The listing builds one solid part. Answer for the finished solid, in the listing's coordinates (mm). A direction names the side the tool comes from. Coordinates: 2 decimals unless noted, no trailing zeros. Write each loop counter-clockwise with the first axis right and the second up, starting at its lowest first coordinate (ties: lowest second). Pieces come first, ordered by that corner, then holes.
(1) The part is cut by section D-D on y = 3.5. Determine the outline of the cut face in (x, z).
(2) The part is cut by section C-C on x = 26. Determine the outline of the cut face in (y, z).
(3) For a pull along X with two mould halves and no side action, classify faces 1 (the flat face through (26, 0.5, 11)), 2 (the cylindrical face through (-28.747, 2.965, 5.121)), 3 (the cylindrical face through (0, 23, 11)) as +X half, -X half, draft (parallel to the pull), parting line (faces both ways), or undercut.
(4) Which of the six approach directions +Z, -Z, +X, -X, +Y, -Y give full straight-line access (tool end or side, diameter ignored) to faces 4 (the flat face through (-28, 5.5, 11)), 5 (the flat face through (28, 5.5, 11)), 6 (the cylindrical face through (0, 18, 11))?
(5) The part is cut by section B-B on y = 17. Determine the outline of the cut face in (x, z).
(6) Given P1, Ø6, axis at x = 29, z = 7.5, coming from the +Y side; P2, Ø12, axis at y = 20, z = 8, coming from the -X side; P3, Ø4.5, axis at x = -26, z = 18, coming from the -Y side; P4, Ø6.5, axis at x = 26, z = 5, coming from the -Y side, each flat-ended and moving along its own axis, determine where each tip first touches the part or whether it passes through.
(7) Straight lines are drawn through the part: line 1 (Z direction, x = -26, y = 2.95); line 2 (X direction, y = 4.5, z = 5.75); line 3 (X direction, y = 8.25, z = 15). For each, find the intervals that lie inside material, in ascending order.
from build123d import *

# Parameters (mm, degrees)
BOSS_EXTRUDE1_DEPTH = 23
SKETCH2_R           = 2.75
CUT_EXTRUDE1_DEPTH  = 47.810789355


with BuildPart() as part:
    # Sketch1 → Boss-Extrude1 (new body)
    with BuildSketch(Plane.XY):
        with BuildLine():
            Line((-17.993054215, 0.5), (-34, 0.5))
            Line((-34, 0.5), (-34, 5.5))
            Line((-34, 5.5), (-22.332711434, 5.5))
            ThreePointArc((-22.332711434, 5.5), (0, 23), (22.332711434, 5.5))
            Line((22.332711434, 5.5), (34, 5.5))
            Line((34, 5.5), (34, 0.5))
            Line((34, 0.5), (17.993054215, 0.5))
            ThreePointArc((17.993054215, 0.5), (0, 18), (-17.993054215, 0.5))
        make_face()
    extrude(amount=BOSS_EXTRUDE1_DEPTH)

    # Sketch2 → Cut-Extrude1 (cut, through all)
    with BuildSketch(Plane.XZ.offset(-0.5)):
        with Locations((-26, 18)):
            Circle(SKETCH2_R)
        with Locations((-26, 5)):
            Circle(SKETCH2_R)
        with Locations((26, 5)):
            Circle(SKETCH2_R)
        with Locations((26, 18)):
            Circle(SKETCH2_R)
    extrude(amount=-CUT_EXTRUDE1_DEPTH, mode=Mode.SUBTRACT)


solid = part.part
Model answer:
1. outline: (-34, 0) - (-17.66, 0) - (-17.66, 23) - (-34, 23) - close; (17.66, 0) - (34, 0) - (34, 23) - (17.66, 23) - close; hole circle Ø5.5 at (-26, 5); hole circle Ø5.5 at (-26, 18); hole circle Ø5.5 at (26, 5); hole circle Ø5.5 at (26, 18)
2. outline: (0.5, 0) - (5.5, 0) - (5.5, 2.25) - (0.5, 2.25) - close; (0.5, 7.75) - (5.5, 7.75) - (5.5, 15.25) - (0.5, 15.25) - close; (0.5, 20.75) - (5.5, 20.75) - (5.5, 23) - (0.5, 23) - close
3. face 1: draft
3. face 2: undercut
3. face 3: parting line
4. face 4: +Z, -Z, -X, +Y
4. face 5: +Z, -Z, +X, +Y
4. face 6: +Z, -Z, -Y
5. outline: (-15.49, 0) - (-5.92, 0) - (-5.92, 23) - (-15.49, 23) - close; (5.92, 0) - (15.49, 0) - (15.49, 23) - (5.92, 23) - close
6. P1: stops at y = 5.5
6. P2: stops at x = -18.25
6. P3: passes through
6. P4: stops at y = 0.5
7. line 1: z = 0 to 2.25, 7.75 to 15.25, 20.75 to 23
7. line 2: x = -34 to -28.65, -23.35 to -17.43, 17.43 to 23.35, 28.65 to 34
7. line 3: x = -21.47 to -16, 16 to 21.47
